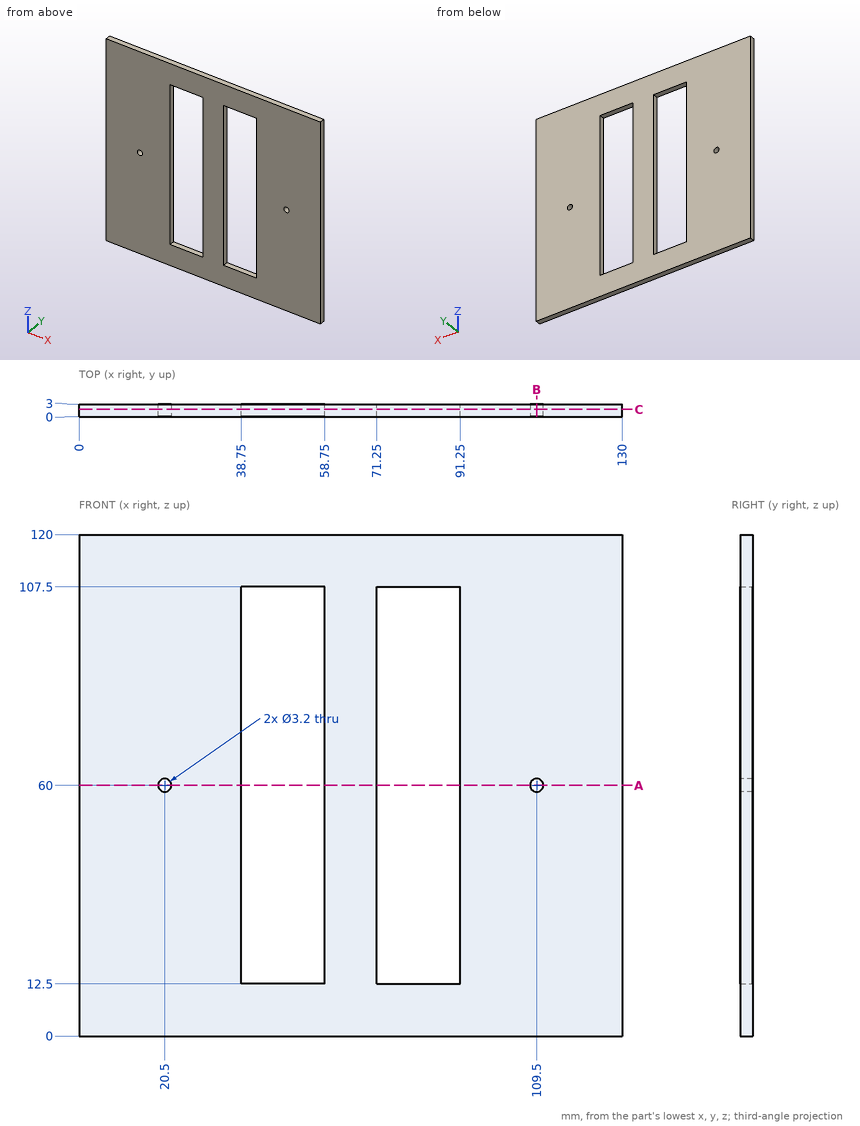
Answer from the drawing. Dimensions are ordinates in mm from the lowest x, y and z of the part. Coordinates: 2 decimals unless noted, no trailing zeros. Write each loop counter-clockwise with the first axis right and the second up, starting at its lowest first coordinate (ties: lowest second). Pieces come first, ordered by that corner, then holes. Notation, with made-up numbers: (28.25, 45) -> (67.25, 45) arc R33 cw to (67.25, 80) -> close; hole circle Ø7 at (4, 36.5). An arc over 180 degrees is marked (long way). One line per question, with ' | ' between items.
1. Section A-A (z = 60) is taken. Determine the outline of the cut face in (x, y), and give its area (3 significant figures).
Verdict:
outline: (0, 0) -> (18.9, 0) -> (18.9, 3) -> (0, 3) -> close; (22.1, 0) -> (38.75, 0) -> (38.75, 3) -> (22.1, 3) -> close; (58.75, 0) -> (71.25, 0) -> (71.25, 3) -> (58.75, 3) -> close; (91.25, 0) -> (107.9, 0) -> (107.9, 3) -> (91.25, 3) -> close; (111.1, 0) -> (130, 0) -> (130, 3) -> (111.1, 3) -> close | area: 251 mm^2
2. Straight lines are drawn through the part: line 1 (X direction, y = 2.8, z = 22); line 2 (Z direction, x = 109.5, y = 0.95); line 3 (Z direction, x = 87, y = 2.85). For each, find the intervals that lie inside material, in ascending order.
Verdict:
line 1: x = 0 to 38.75, 58.75 to 71.25, 91.25 to 130 | line 2: z = 0 to 58.4, 61.6 to 120 | line 3: z = 0 to 12.5, 107.5 to 120
3. Section B-B (x = 109.5) is taken. Determine the outline of the cut face in (y, z), and give its area (3 significant figures).
Verdict:
outline: (0, 0) -> (3, 0) -> (3, 58.4) -> (0, 58.4) -> close; (0, 61.6) -> (3, 61.6) -> (3, 120) -> (0, 120) -> close | area: 350 mm^2
4. Section C-C (y = 1.7) is taken. Determine the outline of the cut face in (x, z), and give its area (3 significant figures).
Verdict:
outline: (0, 0) -> (130, 0) -> (130, 120) -> (0, 120) -> close; hole circle Ø3.2 at (20.5, 60); hole (38.75, 12.5) -> (58.75, 12.5) -> (58.75, 107.5) -> (38.75, 107.5) -> close; hole (71.25, 12.5) -> (91.25, 12.5) -> (91.25, 107.5) -> (71.25, 107.5) -> close; hole circle Ø3.2 at (109.5, 60) | area: 11,800 mm^2
